from build123d import *

# Parameters (mm, degrees)
CROQUIS1_R              = 19.35
SALIENTE_EXTRUIR1_DEPTH = 10
VACIADO1_T              = -2
CORTAR_EXTRUIR1_DEPTH   = 8


with BuildPart() as part:
    # Croquis1 → Saliente-Extruir1 (new body)
    with BuildSketch(Plane.XY):
        Circle(CROQUIS1_R)
    extrude(amount=SALIENTE_EXTRUIR1_DEPTH)

    # Vaciado1
    vaciado1_openings = [part.faces().sort_by_distance(p)[0] for p in [
        (0, 0, 10),
    ]]
    offset(amount=VACIADO1_T, openings=vaciado1_openings, kind=Kind.INTERSECTION)

    # Croquis2 → Cortar-Extruir1 (cut)
    with BuildSketch(Plane.XY.offset(10)):
        with BuildLine():
            Line((5.91867852, 18.42258789), (5.212083976, 16.548615671))
            ThreePointArc((5.212083976, 16.548615671), (11.920626225, 12.366173509), (16.346311037, 5.815549456))
            Line((16.346311037, 5.815549456), (18.195253679, 6.584469877))
            ThreePointArc((18.195253679, 6.584469877), (13.903068898, 14.418007159), (5.91867852, 18.42258789))
        make_face()
    extrude(amount=-CORTAR_EXTRUIR1_DEPTH, mode=Mode.SUBTRACT)


solid = part.part
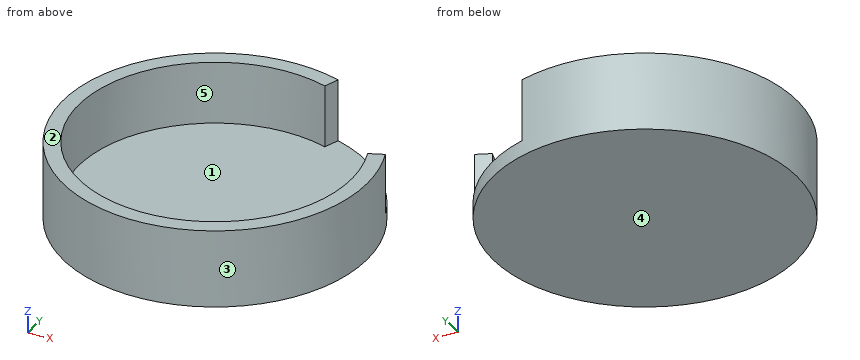
Can you work these out from the model? Positions are in its coordinate system, mm. Face numbers are marked on the shaded views. A direction names the side the tool comes from. Coordinates: 2 decimals unless noted, no trailing zeros. Write each loop counter-clockwise with the first axis right and the second up, starting at its lowest first coordinate (ties: lowest second). Pieces come first, ordered by that corner, then holes.
Q1. Imagine slicing it at A-A, the plane x = 0. List the corners of the cut face in (y, z) for me, plus the area to 3 significant figures.
Results found:
outline: (-19.35, 0) - (19.35, 0) - (19.35, 10) - (17.35, 10) - (17.35, 2) - (-17.35, 2) - (-17.35, 10) - (-19.35, 10) - close
area: 109 mm2
Q2. Please list where these lines run through material, in increasing order: L1, parallel to Y at x = 0, z = 4.75; L2, parallel to Z at x = 1, y = -4.
Results found:
L1: y = -19.35 to -17.35, 17.35 to 19.35
L2: z = 0 to 2
Q3. Which directions (+Z, -Z, +X, -X, +Y, -Y) give clear straight access to the entire face, cutting with the end or side of a thin tool? Please do the marked faces 4 and 5.
Results found:
face 4: -Z, +X, -X, +Y, -Y
face 5: +Z
Q4. For P1, Ø1, axis at y = -8.5, z = 2, coming from the +X side; P2, Ø5, axis at x = 5, z = 8, coming from the +Y side; P3, Ø1.5, axis at x = 7.5, z = 8.5, coming from the +Y side, each with a flat end and sliding along its axis, tell me the tip position at first contact or that it passes through.
Results found:
P1: stops at x = 17.62
P2: stops at y = 19.19
P3: stops at y = -15.26
Q5. Imagine slicing it at C-C, the plane z = 1.25. List the corners of the cut face in (x, y) for me.
Results found:
outline: circle Ø38.7 at (0, 0)
Q6. If we mould it in two halves opening along X, with no side actions, what happens to the marked faces 1, 2 and 3? For each: +X half, -X half, draft (parallel to the pull), parting line (faces both ways), or undercut.
Results found:
face 1: undercut
face 2: draft
face 3: parting line
Q7. Imagine slicing it at D-D, the plane y = 10. List the corners of the cut face in (x, z) for me, plus the area to 3 significant figures.
Results found:
outline: (-16.57, 0) - (16.57, 0) - (16.57, 2) - (-14.18, 2) - (-14.18, 10) - (-16.57, 10) - close
area: 85.4 mm2
